CAD build for the part. Positions are in the model's coordinates, mm. A direction names the side the tool comes from. Give positions to 0.01 mm unless a question says otherwise; leave off trailing zeros.
from build123d import *

# Parameters (mm, degrees)
F0_W     = 2.38125
F0_H     = 6.35
F0_W_2   = 1.3462
F0_W_3   = 6.71068
F0_W_4   = 1.0668
F0_W_5   = 0.8128
F0_W_6   = 0.4064
F0_W_7   = 0.3048
F1_DEPTH = 25.4
F2_DEPTH = 2.54


# Not quite as in the source:
# - ends of sketch curves that miss each other by under 0.0002 mm in the source are joined


with BuildPart() as f1:
    # F0 (on Top) → F1 (new body)
    with BuildSketch(Plane.XY):
        with Locations((-22.328797859, -3.175)):
            Rectangle(F0_W, F0_H)
        with Locations((18.152452141, -3.175)):
            Rectangle(F0_W, F0_H)
        with Locations((-20.465072859, -3.175)):
            Rectangle(F0_W_2, F0_H)
        with Locations((-16.436632859, -3.175)):
            Rectangle(F0_W_3, F0_H)
        with Locations((-12.547892859, -3.175)):
            Rectangle(F0_W_4, F0_H)
        with Locations((-8.659152859, -3.175)):
            Rectangle(F0_W_3, F0_H)
        with Locations((-4.897412859, -3.175)):
            Rectangle(F0_W_5, F0_H)
        with Locations((-1.135672859, -3.175)):
            Rectangle(F0_W_3, F0_H)
        Polygon((2.829267141, 0), (2.219667141, 0), (2.219667141, -6.3499879551), (2.829267141, -6.35), align=None)
        with Locations((6.184607141, -3.175)):
            Rectangle(F0_W_3, F0_H)
        with Locations((9.743147141, -3.175)):
            Rectangle(F0_W_6, F0_H)
        with Locations((13.301687141, -3.175)):
            Rectangle(F0_W_3, F0_H)
        with Locations((16.809427141, -3.175)):
            Rectangle(F0_W_7, F0_H)
    extrude(amount=F1_DEPTH)

    # F0 (on Top) → F2 (join)
    with BuildSketch(Plane.XY):
        with Locations((-22.328797859, -3.175)):
            Rectangle(F0_W, F0_H)
        with Locations((-16.436632859, -3.175)):
            Rectangle(F0_W_3, F0_H)
        with Locations((-8.659152859, -3.175)):
            Rectangle(F0_W_3, F0_H)
        with Locations((-1.135672859, -3.175)):
            Rectangle(F0_W_3, F0_H)
        with Locations((6.184607141, -3.175)):
            Rectangle(F0_W_3, F0_H)
        with Locations((13.301687141, -3.175)):
            Rectangle(F0_W_3, F0_H)
        with Locations((18.152452141, -3.175)):
            Rectangle(F0_W, F0_H)
    extrude(amount=-F2_DEPTH)


solid = f1.part
1. Wall check: line 1 (Z direction, x = -21, y = -4.75). Give the ranges that are in metal, low to high.
2. 3-axis set-ups, long thin cutter, end or side, ignore diameter. For faces 1 (the flat face through (-2, -3, 25.4)), 2 (the flat face through (-12.6, -3.1, 0)): which of +Z, -Z, +X, -X, +Y, -Y reach the whole face in a straight line?
3. Mould opens along X. For faces 3 (the flat face through (2.22, -3, -1)), 4 (the flat face through (19.343, -3, 11)), 5 (the flat face through (-22, -3, -2.54)), 6 (the flat face through (-5.304, -3, -1)) say: released by +X, released by -X, zero draft, split by the parting line, or undercut.
Reported:
1. line 1: z = 0 to 25.4
2. face 1: +Z, +X, -X, +Y, -Y
2. face 2: -Z, +Y, -Y
3. face 3: undercut
3. face 4: released by +X
3. face 5: zero draft
3. face 6: undercut
